Source: CAD feature listing. Evaluate the final solid. Frame: model axes, mm. Give positions to 0.01 mm unless a question says otherwise; leave off trailing zeros. Order: outer loops, then holes, each group sorted by start corner. A loop starts at its lowest first (then second) coordinate and runs counter-clockwise, first axis right, second up. Notation, with made-up numbers: M -12.5,-38 L 23.5,-38 A9 ccw 23.5,-27 Z; hole C -4,55 d6. An arc over 180 degrees is marked long. One line per question, with ' | ' between items. Start each with the question number.
from build123d import *

# Parameters (mm, degrees)
EXTRUDE_1_DEPTH     = 4
SKETCH_3_R          = 1.525
CUT_EXTRUDE_1_DEPTH = 5
SKETCH_4_R          = 14
CUT_EXTRUDE_2_DEPTH = 5
SKETCH_7_R          = 1.525
CUT_EXTRUDE_4_DEPTH = 5
SKETCH_8_W          = 1
SKETCH_8_H          = 57
EXTRUDE_2_DEPTH     = 4
FILLET_1_R          = 2


with BuildPart() as part:
    # 草图1 → 凸台-拉伸1 (new body)
    with BuildSketch(Plane(origin=(0, 0, 0), x_dir=(1, 0, 0), z_dir=(0, 1, 0))):
        with BuildLine():
            ThreePointArc((19.5, 28.5), (-9, 0), (19.5, -28.5))
            Line((19.5, -28.5), (19.5, 28.5))
        make_face()
        with BuildLine():
            Line((19.5, 28.5), (19.5, -28.5))
            ThreePointArc((19.5, -28.5), (39.652543264, -20.152543264), (48, 0))
            ThreePointArc((48, 0), (39.652543264, 20.152543264), (19.5, 28.5))
        make_face()
        with BuildLine():
            Line((-19.5, 28.5), (-19.5, -28.5))
            Line((-19.5, -28.5), (19.5, -28.5))
            ThreePointArc((19.5, -28.5), (-9, 0), (19.5, 28.5))
            Line((19.5, 28.5), (-19.5, 28.5))
        make_face()
    extrude(amount=EXTRUDE_1_DEPTH)

    # 草图3 → 切除-拉伸1 (cut, through all)
    with BuildSketch(Plane(origin=(0, 4, 0), x_dir=(1, 0, 0), z_dir=(0, 1, 0))):
        with Locations((32.935028843, 13.435028843)):
            Circle(SKETCH_3_R)
        with Locations((32.935028843, -13.435028843)):
            Circle(SKETCH_3_R)
        with Locations((6.064971157, -13.435028843)):
            Circle(SKETCH_3_R)
        with Locations((6.064971157, 13.435028843)):
            Circle(SKETCH_3_R)
        with Locations((38.5, 0)):
            Circle(SKETCH_3_R)
        with Locations((19.5, -19)):
            Circle(SKETCH_3_R)
        with Locations((0.5, 0)):
            Circle(SKETCH_3_R)
        with Locations((19.5, 19)):
            Circle(SKETCH_3_R)
    extrude(amount=-CUT_EXTRUDE_1_DEPTH, mode=Mode.SUBTRACT)

    # 草图4 → 切除-拉伸2 (cut, through all)
    with BuildSketch(Plane(origin=(0, 4, 0), x_dir=(1, 0, 0), z_dir=(0, 1, 0))):
        with Locations((19.5, 0)):
            Circle(SKETCH_4_R)
    extrude(amount=-CUT_EXTRUDE_2_DEPTH, mode=Mode.SUBTRACT)

    # 草图7 → 切除-拉伸4 (cut, through all)
    with BuildSketch(Plane.XZ):
        with Locations((-17, 0)):
            Circle(SKETCH_7_R)
        with Locations((-17, 19.5)):
            Circle(SKETCH_7_R)
        with Locations((-17, -19.5)):
            Circle(SKETCH_7_R)
    extrude(amount=-CUT_EXTRUDE_4_DEPTH, mode=Mode.SUBTRACT)

    # 草图8 → 凸台-拉伸2 (add)
    with BuildSketch(Plane(origin=(0, 4, 0), x_dir=(1, 0, 0), z_dir=(0, 1, 0))):
        with Locations((-20, 0)):
            Rectangle(SKETCH_8_W, SKETCH_8_H)
    extrude(amount=-EXTRUDE_2_DEPTH)

    # 圆角1
    fillet_1_edges = [part.edges().sort_by_distance(p)[0] for p in [
        (-20.5, 2, 28.5),
        (-20.5, 2, -28.5),
    ]]
    fillet(fillet_1_edges, radius=FILLET_1_R)


solid = part.part
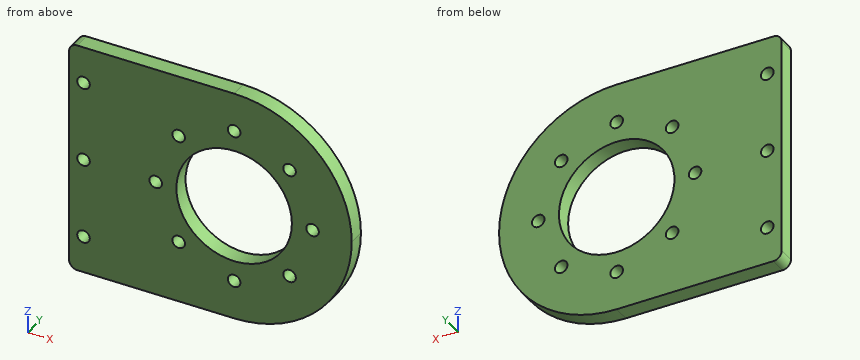
Item 1: Cut plane B-B on x = 0.5. Return the cut outline in (y, z) (3 decimals), and give its area (3 significant figures).
Item 2: Cut plane A-A on x = -17. Return the cut outline in (y, z) (3 decimals), and give its area (3 significant figures).
Item 3: Cut plane D-D on x = 15. Return the cut outline in (y, z).
Item 4: Cut plane C-C on y = 1.25. Count the separate pieces of the cut face and the enclosed holes in it, and give its area (3 significant figures).
Item 5: Pin query (flat end, axial travel): pin 1 Ø1.8 at (x, z) = (19.5, 19) entering from +Y; pin 2 Ø2 at (x, y) = (37.5, 1) entering from -Z. Return the tip coordinate at first contact, or that it passes through.
Item 6: Line query: line 1 (Z direction, x = -17, y = 2.1) (3 decimals); line 2 (Z direction, x = 0.5, y = 1.1) (3 decimals); line 3 (Z direction, x = 19.5, y = 2.1) (3 decimals). Output: solid intervals per line, ascending.
Results are:
1) outline: M 0,-28.5 L 4,-28.5 L 4,-1.525 L 0,-1.525 Z; M 0,1.525 L 4,1.525 L 4,28.5 L 0,28.5 Z | area: 216 mm2
2) outline: M 0,-28.5 L 4,-28.5 L 4,-21.025 L 0,-21.025 Z; M 0,-17.975 L 4,-17.975 L 4,-1.525 L 0,-1.525 Z; M 0,1.525 L 4,1.525 L 4,17.975 L 0,17.975 Z; M 0,21.025 L 4,21.025 L 4,28.5 L 0,28.5 Z | area: 191 mm2
3) outline: M 0,-28.5 L 4,-28.5 L 4,-13.26 L 0,-13.26 Z; M 0,13.26 L 4,13.26 L 4,28.5 L 0,28.5 Z
4) separate pieces: 1 | enclosed holes: 12 | area: 2,860 mm2
5) pin 1: passes through | pin 2: stops at z = -22.87
6) line 1: z = -28.5 to -21.025, -17.975 to -1.525, 1.525 to 17.975, 21.025 to 28.5 | line 2: z = -28.5 to -1.525, 1.525 to 28.5 | line 3: z = -28.5 to -20.525, -17.475 to -14, 14 to 17.475, 20.525 to 28.5
